The listing builds one solid part. Answer for the finished solid, in the listing's coordinates (mm). Face numbers are marked on the shaded views. A direction names the side the tool comes from. Coordinates: 2 decimals unless noted, no trailing zeros. Order: outer loops, then holes, each group sorted by start corner. A loop starts at its lowest first (then second) coordinate and runs counter-clockwise, first axis right, second up. Notation, with made-up numbers: (11, 46.25) - (27, 46.25) arc R23 cw to (27, 78.25) - close; hole circle Ø11 at (-27.75, 32). An arc over 180 degrees is marked (long way). Use a Markdown table: item, result. Add a question column.
Item 1: The part is cut by section D-D, the plane x = -8. Give the vertices of the cut face in (y, z), then the cut area to 3 significant figures.
Item 2: Flat-ended cylindrical pins translate along their axes: P1, Ø1.7, axis at x = -19, y = 37.5, coming from the -Z side; P2, Ø4.5, axis at x = 18.5, y = 61, coming from the -Z side; P3, Ø6, axis at x = -14, z = -8.5, coming from the -Y side; P4, Ø0.6, axis at y = 80, z = -10.5, coming from the +X side. Find the tip coordinate at first contact, or state that the pin passes through.
Item 3: The mould has two halves that part along X. Classify the marked faces 3, 4, 5 and 6: released by +X, released by -X, zero draft, split by the parting line, or undercut.
Item 4: The part is cut by section C-C, the plane z = -16. Give the vertices of the cut face in (x, y).
Item 5: The part is cut by section B-B, the plane y = 26.5. Give the vertices of the cut face in (x, z).
Item 6: For the marked faces 1 and 2, determine the directions among +Z, -Z, +X, -X, +Y, -Y from which every point of the face is accessible in a straight line to the end or side of a thin tool.
Item 7: Find the intervals of material crossed by line 1 along X through (y, z) = (38, 4.5); line 2 along Y through (x, z) = (-21.2, 11); line 3 along Y through (x, z) = (-21, 11), in increasing order.
Item 8: The part is cut by section A-A, the plane y = 10.5. Give the vertices of the cut face in (x, z).
from build123d import *

# Parameters (mm, degrees)
BASE_FLANGE1_DEPTH = 22
CUT_EXTRUDE1_DEPTH = 96.665963068
FILLET1_R          = 2
SKETCH4_R          = 1
CUT_EXTRUDE2_DEPTH = 96.665963068
SKETCH5_W          = 24
SKETCH5_H          = 22
TAB1_DEPTH         = 2
SKETCH6_R          = 0.05
CUT_EXTRUDE3_DEPTH = 10
FILLET2_R          = 5
CHAMFER1_SIZE      = 5
SKETCH7_R          = 5
CUT_EXTRUDE4_DEPTH = 96.665963068


# Sheet-metal steps are written as plain solids
with BuildPart() as part:
    # Sketch1 → Base-Flange1 (new body)
    with BuildSketch(Plane.XY):
        with BuildLine():
            Line((-20.5, 0), (-20.5, 77.50445687))
            ThreePointArc((-20.5, 77.50445687), (-19.914213562, 78.918670432), (-18.5, 79.50445687))
            Line((-18.5, 79.50445687), (18.5, 79.50445687))
            ThreePointArc((18.5, 79.50445687), (19.914213562, 78.918670432), (20.5, 77.50445687))
            Line((20.5, 77.50445687), (20.5, 0))
            Line((20.5, 0), (22.5, 0))
            Line((22.5, 0), (22.5, 77.50445687))
            ThreePointArc((22.5, 77.50445687), (21.328427125, 80.332883995), (18.5, 81.50445687))
            Line((18.5, 81.50445687), (-18.5, 81.50445687))
            ThreePointArc((-18.5, 81.50445687), (-21.328427125, 80.332883995), (-22.5, 77.50445687))
            Line((-22.5, 77.50445687), (-22.5, 0))
            Line((-22.5, 0), (-20.5, 0))
        make_face()
    extrude(amount=BASE_FLANGE1_DEPTH)

    # Sketch3 → Cut-Extrude1 (cut, through all)
    with BuildSketch(Plane.ZY.offset(22.5)):
        with BuildLine():
            Line((7, 0), (15, 0))
            Line((15, 0), (15, 2.5))
            ThreePointArc((15, 2.5), (11, 6.5), (7, 2.5))
            Line((7, 2.5), (7, 0))
        make_face()
    extrude(amount=-CUT_EXTRUDE1_DEPTH, mode=Mode.SUBTRACT)

    # Fillet1
    fillet1_edges = [part.edges().sort_by_distance(p)[0] for p in [
        (21.5, 0, 0),
        (-21.5, 0, 0),
        (21.5, 0, 22),
        (-21.5, 0, 7),
        (-21.5, 0, 15),
        (21.5, 0, 7),
        (21.5, 0, 15),
        (-21.5, 0, 22),
    ]]
    fillet(fillet1_edges, radius=FILLET1_R)

    # Sketch4 → Cut-Extrude2 (cut, through all)
    with BuildSketch(Plane.ZY.offset(22.5)):
        with Locations((19, 2.5)):
            Circle(SKETCH4_R)
        with Locations((16.656854249, 8.156854249)):
            Circle(SKETCH4_R)
        with Locations((11, 10.5)):
            Circle(SKETCH4_R)
        with Locations((5.343145751, 8.156854249)):
            Circle(SKETCH4_R)
        with Locations((3, 2.5)):
            Circle(SKETCH4_R)
    extrude(amount=-CUT_EXTRUDE2_DEPTH, mode=Mode.SUBTRACT)

    # Sketch5 → Tab1 (add)
    with BuildSketch(Plane(origin=(0, 81.50445687, 0), x_dir=(1, 0, 0), z_dir=(0, 1, 0))):
        with Locations((0, 11)):
            Rectangle(SKETCH5_W, SKETCH5_H)
    extrude(amount=-TAB1_DEPTH)

    # Sketch6 → Cut-Extrude3 (cut)
    with BuildSketch(Plane(origin=(0, 81.50445687, 0), x_dir=(1, 0, 0), z_dir=(0, 1, 0))):
        with Locations(Location((0, -7, 0), (0, 0, 270))):
            Circle(SKETCH6_R)
    extrude(amount=-CUT_EXTRUDE3_DEPTH, mode=Mode.SUBTRACT)

    # Fillet2
    fillet2_edges = [part.edges().sort_by_distance(p)[0] for p in [
        (-12, 80.50445687, 0),
        (12, 80.50445687, 0),
    ]]
    fillet(fillet2_edges, radius=FILLET2_R)

    # Chamfer1
    chamfer1_edges = [part.edges().sort_by_distance(p)[0] for p in [
        (-12, 80.50445687, -22),
        (12, 80.50445687, -22),
    ]]
    chamfer(chamfer1_edges, length=CHAMFER1_SIZE)

    # Sketch7 → Cut-Extrude4 (cut, through all)
    with BuildSketch(Plane.ZY.offset(22.5)):
        with Locations((11, 40.5)):
            Circle(SKETCH7_R)
        with Locations((11, 60.5)):
            Circle(SKETCH7_R)
        with Locations((11, 20.5)):
            Circle(SKETCH7_R)
    extrude(amount=-CUT_EXTRUDE4_DEPTH, mode=Mode.SUBTRACT)


solid = part.part
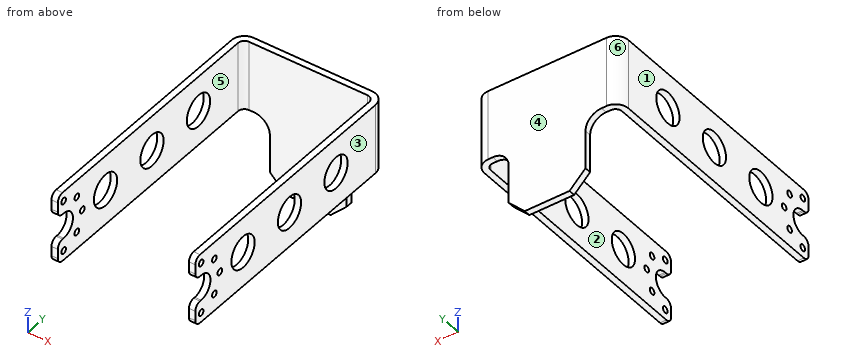
Solution:
| question | item | result |
|---|---|---|
| 1 | outline | (79.5, -21) - (81.5, -21) - (81.5, 22) - (79.5, 22) - close |
| 1 | area | 86.0 mm2 |
| 2 | P1 | passes through |
| 2 | P2 | stops at z = 0 |
| 2 | P3 | stops at y = 79.5 |
| 2 | P4 | stops at x = 12 |
| 3 | face 3 | released by +X |
| 3 | face 4 | zero draft |
| 3 | face 5 | undercut |
| 3 | face 6 | released by -X |
| 4 | outline | (-12, 79.5) - (12, 79.5) - (12, 81.5) - (-12, 81.5) - close |
| 5 | outline | (-22.5, 0) - (-20.5, 0) - (-20.5, 22) - (-22.5, 22) - close; (20.5, 0) - (22.5, 0) - (22.5, 22) - (20.5, 22) - close |
| 6 | face 1 | +Z, -Z, -X, +Y, -Y |
| 6 | face 2 | +Z, -Z, -Y |
| 7 | line 1 | x = -22.5 to -20.5, 20.5 to 22.5 |
| 7 | line 2 | y = 6.5 to 9.5, 11.5 to 15.5, 25.5 to 35.5, 45.5 to 55.5, 65.5 to 80.46 |
| 7 | line 3 | y = 6.5 to 9.5, 11.5 to 15.5, 25.5 to 35.5, 45.5 to 55.5, 65.5 to 80.63 |
| 8 | outline | (-22.5, 0) - (-20.5, 0) - (-20.5, 10) - (-22.5, 10) - close; (-22.5, 12) - (-20.5, 12) - (-20.5, 22) - (-22.5, 22) - close; (20.5, 0) - (22.5, 0) - (22.5, 10) - (20.5, 10) - close; (20.5, 12) - (22.5, 12) - (22.5, 22) - (20.5, 22) - close |
